Build history of the part. All positions in model axes, mm. A direction names the side the tool comes from. Round coordinates to 2 decimals unless told otherwise and drop trailing zeros. Write each loop counter-clockwise with the first axis right and the second up, starting at its lowest first coordinate (ties: lowest second). Pieces come first, ordered by that corner, then holes.
1) Saw through at C-C (y = 25.4). Write the cut outline in (x, z), plus the area to 3 significant figures.
2) Pull direction Z, two halves, no side cores. Call faces 4 (the cylindrical face through (25.06, 15.46, -155.283)), 5 (the flat face through (3, 26, -6.096)), 6 (the flat face through (12.3, 20.5, 0)): +Z half, -Z half, draft (parallel to the pull), parting line (faces both ways), or undercut.
3) Which spindle directions (+Z, -Z, +X, -X, +Y, -Y) get a long thin tool onto all of the face, cutting with end or side? Do faces 1 (the flat face through (24, 26, -6.096)), 2 (the flat face through (20.574, 27.5, -2.3)), 3 (the flat face through (13, 20.32, -88)). Say none if no direction does.
4) Saw through at D-D (x = 10.75). Write the cut outline in (y, z).
5) Saw through at B-B (y = 7.5). Write the cut outline in (x, z) (3 decimals), plus the area to 3 significant figures.
6) Flat gauge pins, fed straight in: pin 1 (10 mm diameter, centred on x = 16.5, z = -81, fed in from -Y); pin 2 (1.7 mm diameter, centred on x = 24, y = 24.5, fed in from -Z); pin 3 (2 mm diameter, centred on x = 23.5, z = -119.5, fed in from +Y). Where does each tip first touch, or does it go through?
7) Saw through at A-A (z = -153.67). Write the cut outline in (x, y) (3 decimals), plus the area to 3 significant figures.
8) Wall check: probe 1 along X at (y, z) = (8, -139.5) (3 decimals); probe 2 along Y at (x, z) = (1.05, -24.13); probe 3 along Z at (x, y) = (25, 25.4). Give the ranges that are in metal, low to high.
from build123d import *

# Parameters (mm, degrees)
BOSS_EXTRUDE2_DEPTH     = 177.8
SKETCH19_R              = 2.032
CUT_EXTRUDE3_DEPTH      = 182.236609161
SKETCH21_W              = 6.096
SKETCH21_H              = 6.096
BOSS_EXTRUDE4_DEPTH     = 5.588
CUT_EXTRUDE4_DEPTH      = 182.233049359
CUT_EXTRUDE4_DEPTH_BACK = 182.233049359
SKETCH22_R              = 2.032


with BuildPart() as part:
    # Sketch2 → Boss-Extrude2 (new body)
    with BuildSketch(Plane.XY):
        with BuildLine():
            Line((0, 0), (0, 22.86))
            Line((0, 22.86), (26.67, 22.86))
            Line((26.67, 22.86), (26.67, 0))
            Line((26.67, 0), (23.495, 0))
            Line((23.495, 0), (23.495, 18.542))
            ThreePointArc((23.495, 18.542), (22.974235857, 19.799235857), (21.717, 20.32))
            Line((21.717, 20.32), (4.953, 20.32))
            ThreePointArc((4.953, 20.32), (3.695764143, 19.799235857), (3.175, 18.542))
            Line((3.175, 18.542), (3.175, 0))
            Line((3.175, 0), (0, 0))
        make_face()
    extrude(amount=-BOSS_EXTRUDE2_DEPTH)

    # Sketch19 → Cut-Extrude3 (cut, through all)
    with BuildSketch(Plane(origin=(0, 0, 0), x_dir=(0, 0, -1), z_dir=(1, 0, 0))):
        with Locations((24.13, 14.224)):
            Circle(SKETCH19_R)
        with Locations((64.77, 14.224)):
            Circle(SKETCH19_R)
        with Locations(Location((113.03, 14.224, 0), (0, 0, 180))):
            Circle(SKETCH19_R)
        with Locations(Location((153.67, 14.224, 0), (0, 0, 180))):
            Circle(SKETCH19_R)
    extrude(amount=CUT_EXTRUDE3_DEPTH, mode=Mode.SUBTRACT)

    # Sketch21 → Boss-Extrude4 (add)
    with BuildSketch(Plane(origin=(0, 22.86, 0), x_dir=(1, 0, 0), z_dir=(0, 1, 0))):
        with Locations((3.048, 3.048)):
            Rectangle(SKETCH21_W, SKETCH21_H)
        with Locations((23.622, 3.048)):
            Rectangle(SKETCH21_W, SKETCH21_H)
    extrude(amount=BOSS_EXTRUDE4_DEPTH)

    # Sketch22 → Cut-Extrude4 (cut, two sides: drawn at the far end of the back side and taken through both)
    with BuildSketch(Plane.ZY.offset(-20.574).offset(-CUT_EXTRUDE4_DEPTH_BACK)):
        with Locations((-3.048, 25.4)):
            Circle(SKETCH22_R)
    extrude(amount=CUT_EXTRUDE4_DEPTH + CUT_EXTRUDE4_DEPTH_BACK, mode=Mode.SUBTRACT)


solid = part.part
Evaluation:
1. outline: (0, -6.1) - (6.1, -6.1) - (6.1, -5.08) - (0, -5.08) - close; (0, -1.02) - (6.1, -1.02) - (6.1, 0) - (0, 0) - close; (20.57, -6.1) - (26.67, -6.1) - (26.67, -5.08) - (20.57, -5.08) - close; (20.57, -1.02) - (26.67, -1.02) - (26.67, 0) - (20.57, 0) - close
1. area: 24.8 mm2
2. face 4: undercut
2. face 5: -Z half
2. face 6: +Z half
3. face 1: -Z, +X, -X, +Y
3. face 2: +Z, -Z, +Y
3. face 3: +Z, -Z, -Y
4. outline: (20.32, -177.8) - (22.86, -177.8) - (22.86, 0) - (20.32, 0) - close
5. outline: (0, -177.8) - (3.175, -177.8) - (3.175, 0) - (0, 0) - close; (23.495, -177.8) - (26.67, -177.8) - (26.67, 0) - (23.495, 0) - close
5. area: 1,130 mm2
6. pin 1: stops at y = 20.32
6. pin 2: stops at z = -6.1
6. pin 3: stops at y = 22.86
7. outline: (0, 0) - (3.175, 0) - (3.175, 12.192) - (0, 12.192) - close; (0, 16.256) - (3.175, 16.256) - (3.175, 18.542) arc R1.778 cw to (4.953, 20.32) - (21.717, 20.32) arc R1.778 cw to (23.495, 18.542) - (23.495, 16.256) - (26.67, 16.256) - (26.67, 22.86) - (0, 22.86) - close; (23.495, 0) - (26.67, 0) - (26.67, 12.192) - (23.495, 12.192) - close
7. area: 172 mm2
8. probe 1: x = 0 to 3.175, 23.495 to 26.67
8. probe 2: y = 0 to 12.19, 16.26 to 22.86
8. probe 3: z = -6.1 to -5.08, -1.02 to 0
